Autodesk Inventor part; units mm, degrees
ref_plane "YZ Plane" through (0, 0, 0) normal (1, 0, 0) x (0, 1, 0)
ref_plane "XZ Plane" through (0, 0, 0) normal (0, 1, 0) x (-1, 0, 0)
ref_plane "XY Plane" through (0, 0, 0) normal (0, 0, 1) x (1, 0, 0)
sketch "Sketch1" plane through (0, 0, 0) normal (0, 1, 0) x (-1, 0, 0)
  line L0 (-37.5, 100) -> (37.5, 100)
  line L1 (37.5, 100) -> (37.5, -100)
  line L2 (37.5, -100) -> (-37.5, -100)
  line L3 (-37.5, -100) -> (-37.5, 100)
  line L4 (-37.5, 100) -> (37.5, -100) construction
  line L5 (37.5, 100) -> (-37.5, -100) construction
  point P0 (0, 0)
  dimension "d0" = 200
  dimension "d1" = 75
extrude "Extrusion1" add sketch "Sketch1" along normal blind 6
sketch "Sketch2" plane through (0, 6, 0) normal (0, 1, 0) x (1, 0, 0)
  circle A0 centre (-24.5, -87.5) radius 3.25
  circle A1 centre (-12, -87.5) radius 3.25
  circle A2 centre (-24.5, 87.5) radius 3.25
  circle A3 centre (-12, 87.5) radius 3.25
  line L0 (-37.5, 100) -> (-37.5, -100)
  line L1 (-37.5, -100) -> (37.5, -100)
  line L2 (37.5, 100) -> (-37.5, 100)
  point P0 (0, 0)
  dimension "d4" = 6.5
  dimension "d5" = 6.5
  dimension "d6" = 12.5
  dimension "d7" = 13
  dimension "d8" = 12.5
  dimension "d9" = 12.5
  dimension "d10" = 6.5
  dimension "d11" = 6.5
  dimension "d12" = 12.5
  dimension "d13" = 13
  dimension "d14" = 12.5
  dimension "d15" = 12.5
extrude "Extrusion2" cut sketch "Sketch2" against normal through all
sketch "Sketch3" plane through (0, 6, 0) normal (0, 1, 0) x (1, 0, 0)
  circle A0 centre (0, -75.052) radius 1.45
  circle A1 centre (20.574, -75.052) radius 1.45
  circle A2 centre (0, -40) radius 1.45
  circle A3 centre (20.574, -40) radius 1.45
  circle A4 centre (0, 40) radius 1.45
  circle A5 centre (20.574, 40) radius 1.45
  circle A6 centre (0, 75.052) radius 1.45
  circle A7 centre (20.574, 75.052) radius 1.45
  point P0 (0, 0)
  dimension "d18" = 2.9
  dimension "d19" = 2.9
  dimension "d20" = 2.9
  dimension "d21" = 2.9
  dimension "d22" = 20.574
  dimension "d23" = 35.052
  dimension "d24" = 35.052
  dimension "d25" = 20.574
  dimension "d26" = 0
  dimension "d27" = 40
  dimension "d28" = 2.9
  dimension "d29" = 2.9
  dimension "d30" = 2.9
  dimension "d31" = 2.9
  dimension "d32" = 20.574
  dimension "d33" = 35.052
  dimension "d34" = 35.052
  dimension "d35" = 20.574
  dimension "d36" = 0
  dimension "d37" = 0
  dimension "d38" = 40
  dimension "d39" = 40
  dimension "d42" = 0
  dimension "d43" = 40
extrude "Extrusion3" cut sketch "Sketch3" against normal through all
properties part number "shelf"
Design review of the part built by this model. Coordinates are the model's own, in mm. Coordinates: 2 decimals unless noted, no trailing zeros. Order: outer loops, then holes, each group sorted by start corner. A loop starts at its lowest first (then second) coordinate and runs counter-clockwise, first axis right, second up. Notation, with made-up numbers: (42.25, 54.5) -> (101.25, 54.5) arc R25 ccw to (101.25, 90.5) -> close; hole circle Ø7 at (-37, 86). An arc over 180 degrees is marked (long way). One line per item, written item: value.
1) Clearance check with a flat-ended pin moving along its axis: P1, Ø4, axis at x = -12, z = -87.5, coming from the -Y side. State where the tip first meets the part, or that it passes through.
Output values:
P1: passes through
2) To check wall thickness, follow probe 1 along Z at (x, y) = (-24.5, 4.05); probe 2 along X at (y, z) = (3.6, -87.5); probe 3 along X at (y, z) = (4.25, -40). State the ranges of each line that lie inside material, in increasing order. Write a range as [from, to].
Output values:
probe 1: z = [-100, -90.75], [-84.25, 84.25], [90.75, 100]
probe 2: x = [-37.5, -27.75], [-21.25, -15.25], [-8.75, 37.5]
probe 3: x = [-37.5, -1.45], [1.45, 19.12], [22.02, 37.5]
3) Draft analysis for pull direction X (two halves, no side actions). For faces 1 (the face through (-12.705, 3.042, -84.327)), 2 (the face through (37.5, 3, -1)), 3 (the face through (-37.5, 3, 1)), 4 (the face through (1, 0, 1)), state which applies: +X half, -X half, draft (parallel to the pull), parting line (faces both ways), or undercut.
Output values:
face 1: undercut
face 2: +X half
face 3: -X half
face 4: draft
4) We need section A-A, the plane x = -12. Give the boundary of the cut face in (y, z), then the cut area to 3 significant figures.
Output values:
outline: (0, -100) -> (6, -100) -> (6, -90.75) -> (0, -90.75) -> close; (0, -84.25) -> (6, -84.25) -> (6, 84.25) -> (0, 84.25) -> close; (0, 90.75) -> (6, 90.75) -> (6, 100) -> (0, 100) -> close
area: 1,120 mm2
5) We need section B-B, the plane z = -87.5. Give the boundary of the cut face in (x, y), then the cut area to 3 significant figures.
Output values:
outline: (-37.5, 0) -> (-27.75, 0) -> (-27.75, 6) -> (-37.5, 6) -> close; (-21.25, 0) -> (-15.25, 0) -> (-15.25, 6) -> (-21.25, 6) -> close; (-8.75, 0) -> (37.5, 0) -> (37.5, 6) -> (-8.75, 6) -> close
area: 372 mm2
